Autodesk Inventor part; units mm, degrees
ref_plane "YZ Plane" through (0, 0, 0) normal (1, 0, 0) x (0, 1, 0)
ref_plane "XZ Plane" through (0, 0, 0) normal (0, 1, 0) x (-1, 0, 0)
ref_plane "XY Plane" through (0, 0, 0) normal (0, 0, 1) x (1, 0, 0)
sketch "Sketch1" plane through (0, 0, 0) normal (0, 1, 0) x (-1, 0, 0)
  line L0 (0, 0) -> (0, -40) construction
  circle A0 centre (0, 0) radius 1.7
  circle A1 centre (0, -40) radius 1.7
  line L1 (-5, -5) -> (5, -5)
  line L2 (5, -5) -> (5, 2)
  line L3 (2, 5) -> (-2, 5)
  line L4 (-5, 2) -> (-5, -5)
  line L5 (-5, -5) -> (5, 5) construction
  line L6 (5, -5) -> (-5, 5) construction
  line L7 (-5, -35) -> (5, -35)
  line L8 (5, -35) -> (5, -42)
  line L9 (2, -45) -> (-2, -45)
  line L10 (-5, -42) -> (-5, -35)
  line L11 (-5, -35) -> (5, -45) construction
  line L12 (5, -35) -> (-5, -45) construction
  arc A2 (5, 2) -> (2, 5) centre (2, 2) ccw
  arc A3 (-2, 5) -> (-5, 2) centre (-2, 2) ccw
  arc A4 (-5, -42) -> (-2, -45) centre (-2, -42) ccw
  arc A5 (2, -45) -> (5, -42) centre (2, -42) ccw
  line L13 (5, -5) -> (5, -35)
  line L14 (-5, -5) -> (-5, -35)
  line L15 (5, -5) -> (-5, -5)
  line L16 (-5, -5) -> (-5, -8)
  line L17 (-5, -8) -> (5, -8)
  line L18 (5, -8) -> (5, -5)
  line L19 (5, -35) -> (-5, -35)
  line L20 (-5, -35) -> (-5, -32)
  line L21 (-5, -32) -> (5, -32)
  line L22 (5, -32) -> (5, -35)
  dimension "d0" = 40
  dimension "d1" = 3.4
  dimension "d2" = 3.4
  dimension "d3" = 10
  dimension "d4" = 10
  dimension "d5" = 10
  dimension "d6" = 10
  dimension "d7" = 3
  dimension "d10" = 3
  dimension "d11" = 3
extrude "Extrusion1" add sketch "Sketch1" along normal blind 3 contours L4 A3 L3 A2 L2 L1 | L7 L8 A5 L9 A4 L10
extrude "Extrusion2" add sketch "Sketch1" along normal blind 16 contours L1 L13 L17 L14 | L21 L13 L7 L14
sketch "Sketch2" plane through (0, 16, 0) normal (0, 1, 0) x (1, 0, 0)
  line L0 (0, 7.9504) -> (0, 32) construction
  line L1 (-5, 32) -> (5, 32)
  circle A0 centre (0, 19.9752) radius 8.65
  line L2 (-5, 5) -> (5, 5)
  line L3 (5, 5) -> (5, 12.9167)
  line L4 (5, 12.9167) -> (-5, 12.9167)
  line L5 (-5, 12.9167) -> (-5, 5)
  line L6 (-5, 42) -> (-5, 35)
  line L7 (-5, 35) -> (5, 35)
  line L8 (5, 35) -> (5, 27.0337)
  line L9 (5, 27.0337) -> (-5, 27.0337)
  line L10 (-5, 27.0337) -> (-5, 35)
  point P0 (0, 0)
  dimension "d14" = 17.3
extrude "Extrusion3" add sketch "Sketch2" along normal blind 5 contours L10 L7 L8 L1 | L1 L8 A0 L10 | A0 L3 L2 L5
sketch "Sketch3" plane through (0, 21, 0) normal (0, 1, 0) x (1, 0, 0)
  line L0 (-5, 5) -> (-5, -2)
  line L1 (5, 35) -> (5, 42)
  line L2 (-5, 5) -> (5, 5)
  line L3 (5, 5) -> (5, 35)
  line L4 (5, 35) -> (-5, 35)
  line L5 (-5, 35) -> (-5, 5)
  point P0 (0, 0)
extrude "Extrusion4" add sketch "Sketch3" along normal blind 3
chamfer "Chamfer2" distance 3 angle 45 4 edges at (0, 16, -8) (0, 16, -32) (0, 3, -35) (0, 3, -5)
sketch "Sketch5" plane through (0, 24, 0) normal (0, 1, 0) x (1, 0, 0)
  line L0 (5, 35) -> (-5, 35) construction
  line L1 (0, 35) -> (0, 5) construction
  line L2 (-5, 5) -> (5, 5) construction
  circle A0 centre (0, 31.5) radius 1.7
  circle A1 centre (0, 8.5) radius 1.7
  point P0 (0, 0)
  dimension "d29" = 3.4
  dimension "d30" = 3.4
  dimension "d31" = 3.5
  dimension "d32" = 3.5
extrude "Extrusion6" cut sketch "Sketch5" against normal blind 8
sketch "Sketch6" plane through (0, 3, 0) normal (0, 1, 0) x (1, 0, 0)
  circle A0 centre (0, 0) radius 5
  circle A1 centre (0, 40) radius 1.7
  circle A2 centre (0, 40) radius 5
  dimension "d35" = 10
  dimension "d36" = 10
extrude "Extrusion7" cut sketch "Sketch6" along normal blind 10
properties part number "Small Gear Bracket"
Geometry: final body of the model. Coordinates: model frame, mm. A direction names the side the tool comes from. Round coordinates to 2 decimals unless told otherwise and drop trailing zeros. Order: outer loops, then holes, each group sorted by start corner. A loop starts at its lowest first (then second) coordinate and runs counter-clockwise, first axis right, second up. Notation, with made-up numbers: (45.5, 86.25) - (71.5, 86.25) arc R30 cw to (71.5, 120.25) - close; hole circle Ø1 at (30, 6.5). An arc over 180 degrees is marked (long way). Write item = value, one per line. Start each with the question number.
Q1. Cut plane C-C on y = 13.5. Return the cut outline in (x, z), and give its area (3 significant figures).
Q2. Ray query, line 1 (Z direction, x = 0, y = 2.3); line 2 (Z direction, x = -2.5, y = 6.5); line 3 (Z direction, x = 0, y = 20.25). Return the intervals inside material, ascending. Write a range as from..to.
Q3. Cut plane B-B on z = 0. Return the cut outline in (x, y), and give its area (3 significant figures).
Q4. Cut plane D-D on z = -31.5. Return the cut outline in (x, y), and give its area (3 significant figures).
Q5. Pull-direction query (Z, two-part tool) for faces 1 (the cylindrical face through (0.37, 1.48, -38.34)), 2 (the flat face through (0, 1, -45)), 3 (the flat face through (0, 6, -32)), 4 (the flat face through (0, 3, 2)); classes: +Z half, -Z half, draft (parallel to the pull), parting line (faces both ways), or undercut.
Q6. Cut plane A-A on y = 2.5. Return the cut outline in (x, z), and give its area (3 significant figures).
Q7. Access query for faces 5 (the cylindrical face through (0, 4, -35)), 6 (the flat face through (0, 21, -20)), 7 (the flat face through (0, 15, -35)), 8 (the flat face through (0, 15, -30)), 9 (the cylindrical face through (-0.37, 20.06, -6.84)). Directions: +Z, -Z, +X, -X, +Y, -Y. A direction counts if a zero-diameter tool reaches every point of the face in a straight line with its end or side. Return the directions, or none.
Q8. Pin query (flat end, axial travel): pin 1 (2 mm diameter, centred on y = 13.5, z = -11.5, fed in from +X); pin 2 (6 mm diameter, centred on x = 1, y = 21.5, fed in from -Z); pin 3 (5 mm diameter, centred on x = 2.5, z = -23.5, fed in from -Y); pin 4 (1 mm diameter, centred on x = 0.5, z = -7.5, fed in from +Y). Return the tip coordinate at first contact, or that it passes through.
Outcome:
q1.outline = (-5, -35) - (5, -35) - (5, -31.5) - (-5, -31.5) - close; (-5, -8.5) - (5, -8.5) - (5, -5) - (-5, -5) - close
q1.area = 70.0 mm^2
q2.line_1 = -45..-41.7, -38.3..-32, -8..-1.7, 1.7..5
q2.line_2 = -35..-32, -8..-5
q2.line_3 = -35..-33.2, -29.8..-28.63, -11.33..-10.2, -6.8..-5
q3.outline = (-5, 0) - (-1.7, 0) - (-1.7, 3) - (-5, 3) - close; (1.7, 0) - (5, 0) - (5, 3) - (1.7, 3) - close
q3.area = 19.8 mm^2
q4.outline = (-5, 13.5) - (5, 13.5) - (5, 24) - (1.7, 24) - (1.7, 16) - (-1.7, 16) - (-1.7, 24) - (-5, 24) - close
q4.area = 77.8 mm^2
q5.face_1 = undercut
q5.face_2 = -Z half
q5.face_3 = undercut
q5.face_4 = draft
q6.outline = (-5, -42) arc R3 ccw to (-2, -45) - (2, -45) arc R3 ccw to (5, -42) - (5, -32) - (-5, -32) - close; (-5, -8) - (5, -8) - (5, 2) arc R3 ccw to (2, 5) - (-2, 5) arc R3 ccw to (-5, 2) - close; hole circle Ø3.4 at (0, -40); hole circle Ø3.4 at (0, 0)
q6.area = 234 mm^2
q7.face_5 = -Z, +Y
q7.face_6 = -Y
q7.face_7 = -Z, +X, -X, +Y
q7.face_8 = +X, -X, -Y
q7.face_9 = +Y
q8.pin_1 = through
q8.pin_2 = -35
q8.pin_3 = 21
q8.pin_4 = 16
